Part model, mm, in its own coordinate system. A direction names the side the tool comes from. Round coordinates to 2 decimals unless told otherwise and drop trailing zeros. Loops run counter-clockwise (first coordinate to the right, second up) from the corner with the lowest first, then second, coordinate; pieces in that order, holes last.
1) Band-saw the part on C-C, the plane y = 9. Write the cut outline in (x, z).
2) Band-saw the part on A-A, the plane z = 0. Write the cut outline in (x, y).
3) Probe line 1 (Y direction, x = 3.75, z = 0.5); line 2 (X direction, y = 3.25, z = -0.5); line 3 (Z direction, x = -4, y = 7). List the from-to ranges inside material, lowest first.
4) Band-saw the part on B-B, the plane y = 2. Write the cut outline in (x, z), then the cut area to 3 significant figures.
5) Drop flat-ended pins along their axis: P1, Ø1.5, axis at x = -1.5, y = 11, coming from the -Z side; P2, Ø6, axis at x = 3, y = 6, coming from the -Z side; P3, Ø2, axis at x = -3.5, y = 7, coming from the +Z side; P4, Ø3, axis at y = 8, z = 5, coming from the -X side. Give the stop position or say it passes through.
6) 3-axis set-ups, long thin cutter, end or side, ignore diameter. For faces 1 (the cylindrical face through (-2.59, 1.83, -4.43)), 2 (the flat face through (-1, 14.486, 0)): which of +Z, -Z, +X, -X, +Y, -Y reach the whole face in a straight line?
from build123d import *

# Parameters (mm, degrees)
FILLET_2_R = 1
FILLET_3_R = 1
FILLET_4_R = 0.5


with BuildPart() as part:
    # 草图1 → 旋转1 (revolve)
    with BuildSketch(Plane.XY, mode=Mode.PRIVATE) as revolve_1_sk:
        Polygon((-1.191258072, 14.485690889), (5, 14.485690889), (5, 4.736615531), (4.320409463, 4.736615531), (4.320409463, 4.0022434), (3.455669657, 4.0022434), (3.455669657, -0.286866039), (-1.191258072, -0.286866039), (-1.191258072, 4.0022434), (-1.191258072, 7.594094591), align=None)
    revolve(revolve_1_sk.sketch.rotate(Axis((-1.191258072, 7.594094591, 0), (0, 1, 0)), 90), axis=Axis((-1.191258072, 7.594094591, 0), (0, 1, 0)))

    # 圆角2
    fillet_2_edges = [part.edges().sort_by_distance(p)[0] for p in [
        (-1.191258072, 14.485690889, 6.191258072),
    ]]
    fillet(fillet_2_edges, radius=FILLET_2_R)

    # 圆角3
    # the kernel refuses this fillet: 1 mm, written as the material it takes off along each edge
    with BuildSketch(Plane(origin=(-1.191258072, 4.736615531, 0), x_dir=(0, 0, -1), z_dir=(1, 0, 0))) as fillet_3_piece_1:
        with BuildLine():
            CenterArc((5.191258072, 0.947279144), FILLET_3_R, 288.687689278, 71.312310722)
            Line((5.511667536, 0), (5.518075725, -0.018945583))
            ThreePointArc((5.518075725, -0.018945583), (5.851462804, -0.02), (6.191258072, -0.02))
            Line((6.191258072, -0.02), (6.211258072, 0))
            Line((6.211258072, 0), (6.211258072, 0.947279144))
            Line((6.211258072, 0.947279144), (6.191258072, 0.947279144))
        make_face()
    revolve(axis=Axis((-1.191258072, 4.736615531, 0), (0, 1, 0)), mode=Mode.SUBTRACT)

    # 圆角4
    fillet_4_edges = [part.edges().sort_by_distance(p)[0] for p in [
        (-1.191258072, 4.0022434, 5.511667536),
    ]]
    fillet(fillet_4_edges, radius=FILLET_4_R)


solid = part.part
Reported:
1. outline: circle Ø12.38 at (-1.19, 0)
2. outline: (-7.38, 5.68) arc R1 ccw to (-6.7, 4.74) - (-6.7, 4.5) arc R0.5 ccw to (-6.2, 4) - (-5.84, 4) - (-5.84, -0.29) - (3.46, -0.29) - (3.46, 4) - (3.82, 4) arc R0.5 ccw to (4.32, 4.5) - (4.32, 4.74) arc R1 ccw to (5, 5.68) - (5, 13.49) arc R1 ccw to (4, 14.49) - (-6.38, 14.49) arc R1 ccw to (-7.38, 13.49) - close
3. line 1: y = 4 to 14.49
3. line 2: x = -5.81 to 3.43
3. line 3: z = -5.52 to 5.52
4. outline: circle Ø9.29 at (-1.19, 0)
4. area: 67.8 mm2
5. P1: stops at z = -6.19
5. P2: stops at z = -6.08
5. P3: stops at z = 6.05
5. P4: stops at x = -6.3
6. face 1: -Y
6. face 2: +Z, -Z, +X, -X, +Y
